Design review of the part built by this model. Coordinates are the model's own, in mm. Give positions to 0.01 mm unless a question says otherwise; leave off trailing zeros. Write each loop counter-clockwise with the first axis right and the second up, starting at its lowest first coordinate (ties: lowest second). Pieces come first, ordered by that corner, then holes. Notation, with made-up numbers: (14, 58.5) -> (43, 58.5) arc R21 ccw to (43, 75.5) -> close; hole circle Ø9 at (25.25, 45.25). An arc over 180 degrees is marked (long way). Answer as a JSON object with one key per item and string values.
```python
from build123d import *

# Parameters (mm, degrees)
BASPROSKE_W         = 4
BASPROSKE_H         = 6
TOOTHCUT_DEPTH      = 10.38083152
TEETHCUTS_COUNT     = 10
BORSKE_R            = 1
BORE_DEPTH          = 50.0000508
SKETCH_1_R          = 1.25
CUT_EXTRUDE_1_DEPTH = 10


with BuildPart() as part:
    # BasProSke → Base-Revolve (revolve)
    with BuildSketch(Plane(origin=(0, 0, 0), x_dir=(1, 0, 0), z_dir=(0, 1, 0)), mode=Mode.PRIVATE) as base_revolve_sk:
        with Locations((2, 3)):
            Rectangle(BASPROSKE_W, BASPROSKE_H)
    revolve(base_revolve_sk.sketch.rotate(Axis((-10, 0, 0), (1, 0, 0)), 180), axis=Axis((-10, 0, 0), (1, 0, 0)))

    # TooCutSke → ToothCut (cut, through all)
    with BuildSketch(Plane(origin=(0, 0, 0), x_dir=(0, 0, -1), z_dir=(1, 0, 0))):
        with BuildLine():
            ThreePointArc((0.59278292, 3.701838653), (0, 3.749), (-0.59278292, 3.701838653))
            ThreePointArc((-0.59278292, 3.701838653), (-0.846593509, 4.924114224), (-1.775771316, 5.757784417))
            ThreePointArc((-1.775771316, 5.757784417), (0, 6.0254), (1.775771316, 5.757784417))
            ThreePointArc((1.775771316, 5.757784417), (0.846593509, 4.924114224), (0.59278292, 3.701838653))
        make_face()
    toothcut = extrude(amount=TOOTHCUT_DEPTH, mode=Mode.SUBTRACT)

    # TeethCuts: ToothCut ×10 about axis
    teethcuts_axis = Axis((0, 0, 0), (1, 0, 0))
    for i in range(1, TEETHCUTS_COUNT):
        add(toothcut.rotate(teethcuts_axis, i * 360 / TEETHCUTS_COUNT), mode=Mode.SUBTRACT)

    # BorSke → Bore (cut, symmetric)
    with BuildSketch(Plane(origin=(0, 0, 0), x_dir=(0, 0, -1), z_dir=(1, 0, 0))):
        with Locations(Location((0, 0, 0), (0, 0, 180))):
            Circle(BORSKE_R)
    extrude(amount=BORE_DEPTH, both=True, mode=Mode.SUBTRACT)

    # 草图1 → 切除-拉伸1 (cut)
    with BuildSketch(Plane(origin=(4, 0, 0), x_dir=(0, 0, -1), z_dir=(1, 0, 0))):
        Circle(SKETCH_1_R)
    extrude(amount=-CUT_EXTRUDE_1_DEPTH, mode=Mode.SUBTRACT)


solid = part.part
```
(1) For line 1 along Y through (x, z) = (0.95, 0); line 2 along Y through (x, z) = (2.95, 4.75); line 3 along Z through (x, y) = (1.2, -3.25), list the stretches that pass through material, from the lowest coordinate up.
Here are the results:
{"line 1": "y = -3.75 to -1.25, 1.25 to 3.75", "line 2": "y = -3.63 to -2.82, -0.75 to 0.75, 2.82 to 3.63", "line 3": "z = -4.89 to -3.18, -1.87 to 1.87, 3.18 to 4.89"}
(2) We need section C-C, the plane z = 4.5. State the section outline as (x, y) points, then the cut area to 3 significant figures.
Here are the results:
{"outline": "(0, -3.66) -> (4, -3.66) -> (4, -2.42) -> (0, -2.42) -> close; (0, -0.76) -> (4, -0.76) -> (4, 0.76) -> (0, 0.76) -> close; (0, 2.42) -> (4, 2.42) -> (4, 3.66) -> (0, 3.66) -> close", "area": "16.0 mm²"}
(3) We need section B-B, the plane y = 4. State the section outline as (x, z) points, then the cut area to 3 significant figures.
Here are the results:
{"outline": "(0, -2.1) -> (4, -2.1) -> (4, -0.58) -> (0, -0.58) -> close; (0, 0.58) -> (4, 0.58) -> (4, 2.1) -> (0, 2.1) -> close", "area": "12.1 mm²"}
(4) Clearance check with flat-ended pins moving along their axes: pin 1 (2 mm diameter, centred on x = 3, z = 3.5, fed in from -Y); pin 2 (1.5 mm diameter, centred on x = 1, y = -3.5, fed in from +Z). State where each tip first meets the part, or that it passes through.
Here are the results:
{"pin 1": "stops at y = -3.66", "pin 2": "stops at z = 4.92"}
(5) The part is to be moulded in two halves that separate along Z. For faces 1 (the flat face through (0, -0.1, 1.4)), 2 (the cylindrical face through (1.972, 4.892, 0.829)), say which applies: +Z half, -Z half, draft (parallel to the pull), parting line (faces both ways), or undercut.
Here are the results:
{"face 1": "draft", "face 2": "undercut"}
(6) We need section A-A, the plane z = 0. State the section outline as (x, y) points.
Here are the results:
{"outline": "(0, -3.75) -> (4, -3.75) -> (4, -1.25) -> (0, -1.25) -> close; (0, 1.25) -> (4, 1.25) -> (4, 3.75) -> (0, 3.75) -> close"}
